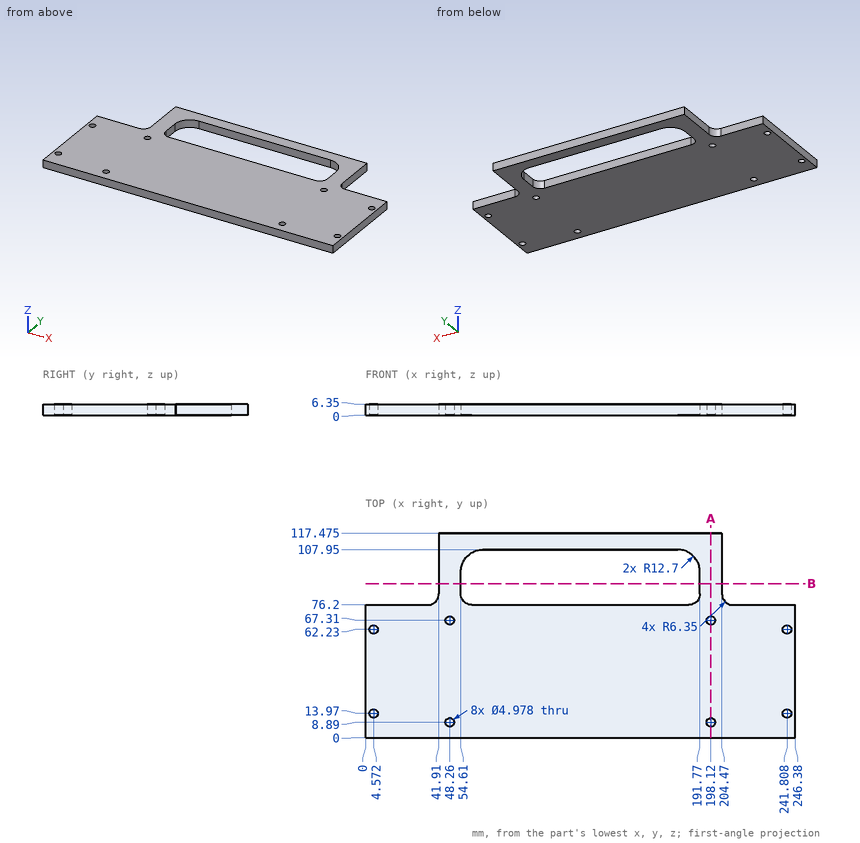
The figure shows three views and two pictorial views of one solid part (mm, origin at its lowest corner). Answer the questions. Coordinates: 2 decimals unless noted, no trailing zeros. Write each loop counter-clockwise with the first axis right and the second up, starting at its lowest first coordinate (ties: lowest second). Pieces come first, ordered by that corner, then holes.
1. The part is cut by section A-A, the plane x = 198.12. State how many separate pieces and enclosed holes the cut face has, and give its area (3 significant figures).
Results list:
separate pieces: 3
enclosed holes: 0
area: 683 mm2
2. Consider line 1 along Y through (x, z) = (48.26, 3) (1 decimal); line 2 along X through (y, z) = (92, 3.75); line 3 along Y through (x, z) = (231, 4.25). Determine where each line is inside the solid, lowest interval first.
Results list:
line 1: y = 0 to 6.4, 11.4 to 64.8, 69.8 to 117.5
line 2: x = 41.91 to 54.61, 191.77 to 204.47
line 3: y = 0 to 76.2
3. Flat-ended cylindrical pins translate along their axes: pin 1 (1.9 mm diameter, centred on y = 100, z = 2, fed in from +X); pin 2 (3 mm diameter, centred on x = 221, z = 4, fed in from +Y). Find the tip coordinate at first contact, or state that the pin passes through.
Results list:
pin 1: stops at x = 204.47
pin 2: stops at y = 76.2
4. The part is cut by section B-B, the plane y = 88.5. Write down the section's boundary in (x, z).
Results list:
outline: (41.91, 0) - (54.61, 0) - (54.61, 6.35) - (41.91, 6.35) - close; (191.77, 0) - (204.47, 0) - (204.47, 6.35) - (191.77, 6.35) - close
